The listing builds one solid part. Answer for the finished solid, in the listing's coordinates (mm). Face numbers are marked on the shaded views. Give positions to 0.01 mm unless a question says otherwise; leave off trailing zeros. Write each loop counter-clockwise with the first axis right and the second up, starting at its lowest first coordinate (ties: lowest second). Pieces come first, ordered by that corner, then holes. Notation, with made-up numbers: (18, -12) - (40, -12) arc R33 ccw to (40, 25) - close; hole circle Ø1 at (70.25, 73). An arc over 180 degrees is marked (long way). One line per item, written item: value. Start each with the question number.
from build123d import *

# Parameters (mm, degrees)
SKETCH1_R           = 5.018077717
SKETCH1_R_2         = 5.15
SKETCH1_R_3         = 3.225
SKETCH1_R_4         = 2.5
BOSS_EXTRUDE1_DEPTH = 5


with BuildPart() as part:
    # Sketch1 → Boss-Extrude1 (new body)
    with BuildSketch(Plane.XY):
        with BuildLine():
            Line((4.242424242, -15), (35.242424242, -15))
            ThreePointArc((35.242424242, -15), (38.070851367, -16.171572875), (39.242424242, -19))
            Line((39.242424242, -19), (39.242424242, -23))
            ThreePointArc((39.242424242, -23), (39.82821068, -24.414213562), (41.242424242, -25))
            Line((41.242424242, -25), (57.242424242, -25))
            ThreePointArc((57.242424242, -25), (58.656637805, -24.414213562), (59.242424242, -23))
            Line((59.242424242, -23), (59.242424242, -7))
            ThreePointArc((59.242424242, -7), (58.656637805, -5.585786438), (57.242424242, -5))
            Line((57.242424242, -5), (35.792732382, -5))
            ThreePointArc((35.792732382, -5), (17.638610474, 0.120331449), (4.778243752, 13.91891486))
            ThreePointArc((4.778243752, 13.91891486), (4.04159661, 14.708483204), (3.001844168, 15))
            Line((3.001844168, 15), (-13.757575758, 15))
            ThreePointArc((-13.757575758, 15), (-15.17178932, 15.585786438), (-15.757575758, 17))
            Line((-15.757575758, 17), (-15.757575758, 23))
            ThreePointArc((-15.757575758, 23), (-16.343362195, 24.414213562), (-17.757575758, 25))
            Line((-17.757575758, 25), (-33.757575758, 25))
            ThreePointArc((-33.757575758, 25), (-35.17178932, 24.414213562), (-35.757575758, 23))
            Line((-35.757575758, 23), (-35.757575758, -23))
            ThreePointArc((-35.757575758, -23), (-35.17178932, -24.414213562), (-33.757575758, -25))
            Line((-33.757575758, -25), (-17.757575758, -25))
            ThreePointArc((-17.757575758, -25), (-16.343362195, -24.414213562), (-15.757575758, -23))
            Line((-15.757575758, -23), (-15.757575758, -19))
            ThreePointArc((-15.757575758, -19), (-14.586002882, -16.171572875), (-11.757575758, -15))
            Line((-11.757575758, -15), (4.242424242, -15))
        make_face()
        with Locations((45.944077131, -15)):
            Circle(SKETCH1_R, mode=Mode.SUBTRACT)
        with Locations((-27.490266303, -15)):
            Circle(SKETCH1_R_2, mode=Mode.SUBTRACT)
        with Locations((-27.490266303, 15)):
            Circle(SKETCH1_R_3, mode=Mode.SUBTRACT)
        with Locations((-2.490266303, 0)):
            Circle(SKETCH1_R_4, mode=Mode.SUBTRACT)
    extrude(amount=BOSS_EXTRUDE1_DEPTH)


solid = part.part
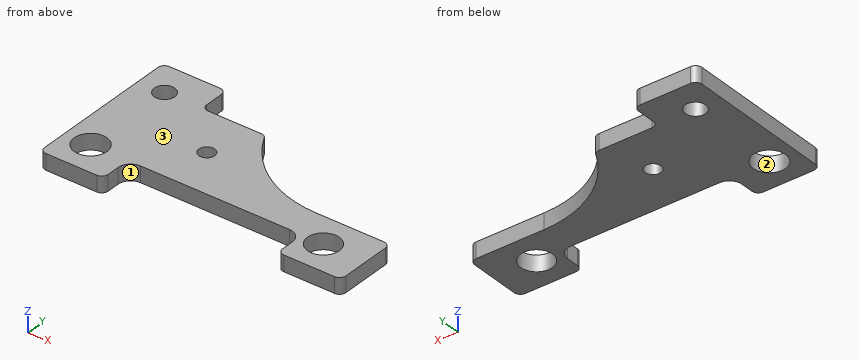
Item 1: Find section B-B on y = -13.5. Determine the outline of the cut face in (x, z).
Item 2: Find section D-D on x = 38. Determine the outline of the cut face in (y, z), plus the area to 3 significant figures.
Item 3: Find section A-A on z = 1.1. Determine the outline of the cut face in (x, y) (3 decimals), plus the area to 3 significant figures.
Item 4: The mould has two halves that part along Y. Classify the marked faces 1, 2 and 3: +Y half, -Y half, draft (parallel to the pull), parting line (faces both ways), or undercut.
Item 5: Find section C-C on y = 0. Determine the outline of the cut face in (x, z), plus the area to 3 significant figures.
Item 6: Straight lines are drawn through the part: line 1 along Y through (x, z) = (-25, 1.8); line 2 along Y through (x, z) = (-25.5, 0.75); line 3 along X through (y, z) = (-14, 0.85). For each, find the intervals that lie inside material, in ascending order.
Item 7: Each of these flat-tipped pins is pushed along its axis until it touches: pin 1 Ø1.5 at (x, z) = (-3.5, 3) entering from +Y; pin 2 Ø2 at (x, z) = (36, 1) entering from +Y; pin 3 Ø3 at (x, y) = (-2.49, 0) entering from -Z. Where does it stop, or does it pass through?
Values:
1. outline: (-35.76, 0) - (-32.42, 0) - (-32.42, 5) - (-35.76, 5) - close; (-22.56, 0) - (41.16, 0) - (41.16, 5) - (-22.56, 5) - close; (50.73, 0) - (59.24, 0) - (59.24, 5) - (50.73, 5) - close
2. outline: (-16.1, 0) - (-5, 0) - (-5, 5) - (-16.1, 5) - close
2. area: 55.5 mm^2
3. outline: (-35.758, -23) arc R2 ccw to (-33.758, -25) - (-17.758, -25) arc R2 ccw to (-15.758, -23) - (-15.758, -19) arc R4 cw to (-11.758, -15) - (35.242, -15) arc R4 cw to (39.242, -19) - (39.242, -23) arc R2 ccw to (41.242, -25) - (57.242, -25) arc R2 ccw to (59.242, -23) - (59.242, -7) arc R2 ccw to (57.242, -5) - (35.793, -5) arc R35 cw to (4.778, 13.919) arc R2 ccw to (3.002, 15) - (-13.758, 15) arc R2 cw to (-15.758, 17) - (-15.758, 23) arc R2 ccw to (-17.758, 25) - (-33.758, 25) arc R2 ccw to (-35.758, 23) - close; hole circle Ø10.3 at (-27.49, -15); hole circle Ø6.45 at (-27.49, 15); hole circle Ø5 at (-2.49, 0); hole circle Ø10.036 at (45.944, -15)
3. area: 2,320 mm^2
4. face 1: -Y half
4. face 2: undercut
4. face 3: draft
5. outline: (-35.76, 0) - (-4.99, 0) - (-4.99, 5) - (-35.76, 5) - close; (0.01, 0) - (17.84, 0) - (17.84, 5) - (0.01, 5) - close
5. area: 243 mm^2
6. line 1: -25 to -19.51, -10.49 to 12.95, 17.05 to 25
6. line 2: -25 to -19.75, -10.25 to 12.46, 17.54 to 25
6. line 3: -35.76 to -32.54, -22.44 to 41.03, 50.86 to 59.24
7. pin 1: y = 15
7. pin 2: y = -4.99
7. pin 3: through
